from build123d import *

# Parameters (mm, degrees)
F2_R     = 1.25
F3_DEPTH = 14


with BuildPart() as f1:
    # F0 (on Front) → F1 (revolve)
    with BuildSketch(Plane.XZ):
        Polygon((-5, 0), (-5, 14), (-7, 14), (-7, 4), (-11, 4), (-11, 0), align=None)
    revolve(axis=Axis((0, 0, -1.594857), (0, 0, -1)))

    # F2 (on face) → F3 (cut)
    with BuildSketch(Plane(origin=(0, 0, 0), x_dir=(1, 0, 0), z_dir=(0, 0, -1))):
        with Locations((0, 8)):
            Circle(F2_R)
        with Locations((-8, 0)):
            Circle(F2_R)
        with Locations((8, 0)):
            Circle(F2_R)
        with Locations((0, -8)):
            Circle(F2_R)
    extrude(amount=-F3_DEPTH, mode=Mode.SUBTRACT)


solid = f1.part
Input: part model. Units: mm. Frame: model coordinates. A direction names the side the tool comes from. Give positions to 0.01 mm unless a question says otherwise; leave off trailing zeros. Write each loop counter-clockwise with the first axis right and the second up, starting at its lowest first coordinate (ties: lowest second). Pieces come first, ordered by that corner, then holes.
Q1. First-contact query: P1, Ø1, axis at x = -7, y = -2, coming from the +Z side; P2, Ø5, axis at y = -6.5, z = 10.5, coming from the +X side; P3, Ø9, axis at x = 0, y = 0, coming from the +Z side; P4, Ø6, axis at x = -6.5, z = 4, coming from the -Y side. Flat tips, straight axial feed; report the tip coordinate or a pass-through.
Q2. Section C-C, the plane x = -8.5. Output: boundary loops of the cut face in (y, z).
Q3. Section A-A, the plane y = 0. Output: boundary loops of the cut face in (x, z), plus the area to 3 significant figures.
Q4. Section D-D, the plane y = 3.5. Output: boundary loops of the cut face in (x, z).
Q5. Pull-direction query (X, two-part tool) for faces 4 (the face through (4.9, 5, 8.9)), 5 (the face through (1.08, -4.88, 7.1)), 6 (the face through (7, -2, 4)); classes: pulls with the +X half, pulls with the -X half, needs draft (parallel to the pull), parting line crosses it, or undercut.
Q6. Material intervals for probe 1 along Y at (x, z) = (0, 10.25); probe 2 along X at (y, z) = (8, 3.25); probe 3 along Z at (x, y) = (4.25, 5.75), sorted ascending.
Q7. Set-up query: faces 1 (the face through (-5, 4.9, 8.9)), 2 (the face through (5, -4.9, 8.9)), 3 (the face through (-4.9, -5, 8.9)). Return all of +Z, -Z, +X, -X, +Y, -Y with unobstructed straight access to the full face (end or side cutting, diameter ignored); none if empty.
Q8. Section B-B, the plane z = 11. Output: boundary loops of the cut face in (x, y).
Filled in:
1. P1: stops at z = 14
1. P2: stops at x = 5.74
1. P3: passes through
1. P4: stops at y = -10.43
2. outline: (-6.98, 0) - (-1.15, 0) - (-1.15, 4) - (-6.98, 4) - close; (1.15, 0) - (6.98, 0) - (6.98, 4) - (1.15, 4) - close
3. outline: (-11, 0) - (-9.25, 0) - (-9.25, 4) - (-11, 4) - close; (-6.75, 0) - (-5, 0) - (-5, 14) - (-6.75, 14) - close; (5, 0) - (6.75, 0) - (6.75, 14) - (5, 14) - close; (9.25, 0) - (11, 0) - (11, 4) - (9.25, 4) - close
3. area: 63.0 mm2
4. outline: (-10.43, 0) - (-3.57, 0) - (-3.57, 14) - (-6.06, 14) - (-6.06, 4) - (-10.43, 4) - close; (3.57, 0) - (10.43, 0) - (10.43, 4) - (6.06, 4) - (6.06, 14) - (3.57, 14) - close
5. face 4: pulls with the +X half
5. face 5: undercut
5. face 6: needs draft
6. probe 1: y = -6.75 to -5, 5 to 6.75
6. probe 2: x = -7.55 to -1.25, 1.25 to 7.55
6. probe 3: z = 0 to 4
7. face 1: +Z, -X, +Y
7. face 2: +Z, +X, -Y
7. face 3: +Z, -X, -Y
8. outline: (-6.96, -0.7) arc R7 ccw to (-0.7, -6.96) arc R1.25 cw to (0.7, -6.96) arc R7 ccw to (6.96, -0.7) arc R1.25 cw to (6.96, 0.7) arc R7 ccw to (0.7, 6.96) arc R1.25 cw to (-0.7, 6.96) arc R7 ccw to (-6.96, 0.7) arc R1.25 cw to start; hole circle Ø10 at (0, 0)
